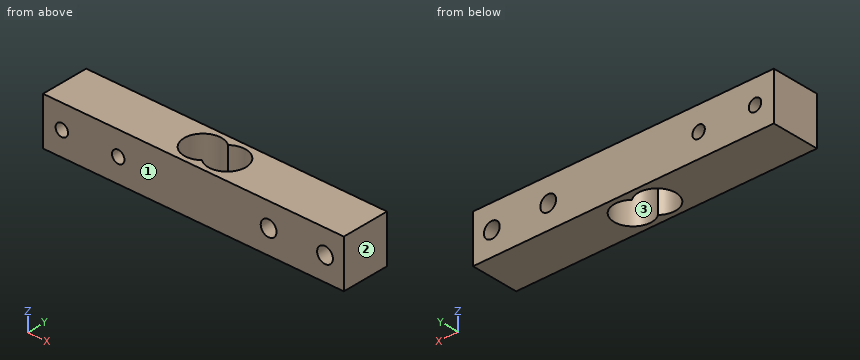
from build123d import *

# Parameters (mm, degrees)
CROQUIS1_W                                 = 80
CROQUIS1_H                                 = 12.7
SALIENTE_EXTRUIR1_DEPTH                    = 12.7
PERFORADOR_PARA_ROSCAR_PARA_MACHO_DE_ROS_D = 3.3
PERFORADOR_PARA_ROSCAR_PARA_MACHO_DE_2_D   = 4.2


with BuildPart() as part:
    # Croquis1 → Saliente-Extruir1 (new body)
    with BuildSketch(Plane.XY):
        Rectangle(CROQUIS1_W, CROQUIS1_H)
        with BuildLine():
            ThreePointArc((0, 3.841213022), (-8.200794046, 0), (0, -3.841213022))
            ThreePointArc((0, -3.841213022), (8.200794046, 0), (0, 3.841213022))
        make_face(mode=Mode.SUBTRACT)
    extrude(amount=SALIENTE_EXTRUIR1_DEPTH)

    # Perforador para roscar para macho de ros (through all)
    with Locations(Plane(origin=(0, 6.35, 0), x_dir=(1, 0, 0), z_dir=(0, 1, 0))):
        with Locations((-35, -6.35), (-20, -6.35)):
            Hole(PERFORADOR_PARA_ROSCAR_PARA_MACHO_DE_ROS_D / 2)

    # Perforador para roscar para macho de 2 (through all)
    with Locations(Plane(origin=(0, 6.35, 0), x_dir=(1, 0, 0), z_dir=(0, 1, 0))):
        with Locations((35, -6.35), (20, -6.35)):
            Hole(PERFORADOR_PARA_ROSCAR_PARA_MACHO_DE_2_D / 2)


solid = part.part
The listing builds one solid part. Answer for the finished solid, in the listing's coordinates (mm). Face numbers are marked on the shaded views. Coordinates: 2 decimals unless noted, no trailing zeros. Order: outer loops, then holes, each group sorted by start corner. A loop starts at its lowest first (then second) coordinate and runs counter-clockwise, first axis right, second up. Notation, with made-up numbers: M -9,-5 L 29,-5 A19 cw 29,6 Z; hole C 20.5,27.25 d11. An arc over 180 degrees is marked long. Use CSV: the item, a comma, the result in double quotes.
Q1. Straight lines are drawn through the part: L1, parallel to Z at x = -35, y = -0.75; L2, parallel to X at y = 5.5, z = 6.25; L3, parallel to X at y = 0.25, z = 4. For each, find the intervals that lie inside material, in ascending order.
Here are the results:
L1,"0 to 4.7, 8 to 12.7"
L2,"-40 to -36.65, -33.35 to -21.65, -18.35 to 17.9, 22.1 to 32.9, 37.1 to 40"
L3,"-40 to -8.19, 8.19 to 40"
Q2. Section B-B (x = -20) is taken. Determine the outline of the cut face in (y, z), then the cut area to 3 significant figures.
Here are the results:
outline,"M -6.35,0 L 6.35,0 L 6.35,4.7 L -6.35,4.7 Z; M -6.35,8 L 6.35,8 L 6.35,12.7 L -6.35,12.7 Z"
area,"119 mm2"
Q3. Determine the mould class of the marked faces 1, 2 and 3 for opening direction Y: pulls with the +Y half, pulls with the -Y half, needs draft (parallel to the pull), parting line crosses it, or undercut.
Here are the results:
face 1,"pulls with the -Y half"
face 2,"needs draft"
face 3,"undercut"
Q4. Section C-C (z = 6.35) is taken. Determine the outline of the cut face in (x, y), then the cut area to 3 significant figures.
Here are the results:
outline,"M -40,-6.35 L -36.65,-6.35 L -36.65,6.35 L -40,6.35 Z; M -33.35,-6.35 L -21.65,-6.35 L -21.65,6.35 L -33.35,6.35 Z; M -18.35,-6.35 L 17.9,-6.35 L 17.9,6.35 L -18.35,6.35 Z; M 22.1,-6.35 L 32.9,-6.35 L 32.9,6.35 L 22.1,6.35 Z; M 37.1,-6.35 L 40,-6.35 L 40,6.35 L 37.1,6.35 Z; hole M 0,-3.84 A5 ccw long 0,3.84 A5 ccw long Z"
area,"688 mm2"
Q5. Section A-A (y = 0) is taken. Determine the outline of the cut face in (x, z).
Here are the results:
outline,"M -40,0 L -8.2,0 L -8.2,12.7 L -40,12.7 Z; M 8.2,0 L 40,0 L 40,12.7 L 8.2,12.7 Z; hole C -35,6.35 d3.3; hole C -20,6.35 d3.3; hole C 20,6.35 d4.2; hole C 35,6.35 d4.2"
Q6. Section D-D (x = -2.5) is taken. Determine the outline of the cut face in (y, z).
Here are the results:
outline,"M -6.35,0 L -4.95,0 L -4.95,12.7 L -6.35,12.7 Z; M 4.95,0 L 6.35,0 L 6.35,12.7 L 4.95,12.7 Z"
